Autodesk Inventor part; units mm, degrees
ref_plane "YZ Plane" through (0, 0, 0) normal (1, 0, 0) x (0, 1, 0)
ref_plane "XZ Plane" through (0, 0, 0) normal (0, 1, 0) x (-1, 0, 0)
ref_plane "XY Plane" through (0, 0, 0) normal (0, 0, 1) x (1, 0, 0)
sketch "Sketch1" plane through (0, 0, 0) normal (0, 0, 1) x (1, 0, 0)
  line L0 (-52.5, -20) -> (52.5, -20)
  line L1 (52.5, 20) -> (-52.5, 20)
  line L2 (-52.5, -20) -> (52.5, 20) construction
  line L3 (52.5, -20) -> (-52.5, 20) construction
  line L4 (-50, 17.5) -> (50, 17.5)
  line L5 (50, -17.5) -> (-50, -17.5)
  line L6 (-50, 17.5) -> (50, -17.5) construction
  line L7 (50, 17.5) -> (-50, -17.5) construction
  line L8 (60.5, 0) -> (60.5, 8)
  line L9 (60.5, 8) -> (52.5, 20)
  line L10 (60.5, 0) -> (60.5, -8)
  line L11 (60.5, -8) -> (52.5, -20)
  line L12 (50, -17.5) -> (56.5426, -7.6861)
  line L13 (56.5426, -7.6861) -> (56.5426, 7.6861)
  line L14 (56.5426, 7.6861) -> (50, 17.5)
  line L15 (0, 0) -> (0, 38.4543) construction
  line L16 (-60.5, 0) -> (-60.5, 8)
  line L17 (-60.5, 8) -> (-52.5, 20)
  line L18 (-60.5, 0) -> (-60.5, -8)
  line L19 (-60.5, -8) -> (-52.5, -20)
  line L20 (-50, -17.5) -> (-56.5426, -7.6861)
  line L21 (-56.5426, -7.6861) -> (-56.5426, 7.6861)
  line L22 (-56.5426, 7.6861) -> (-50, 17.5)
  dimension "d0" = 105
  dimension "d1" = 40
  dimension "d2" = 100
  dimension "d3" = 35
  dimension "d5" = 8
  dimension "d6" = 8
extrude "Extrusion1" add sketch "Sketch1" along normal blind 120
sketch "Sketch2" plane through (0, 0, 120) normal (0, 0, 1) x (1, 0, 0)
  line L0 (-56.5426, 7.6861) -> (-50, 17.5)
  line L1 (-50, 17.5) -> (50, 17.5)
  line L2 (50, 17.5) -> (56.5426, 7.6861)
  line L3 (56.5426, 7.6861) -> (56.5426, -7.6861)
  line L4 (56.5426, -7.6861) -> (50, -17.5)
  line L5 (50, -17.5) -> (-50, -17.5)
  line L6 (-50, -17.5) -> (-56.5426, -7.6861)
  line L7 (-56.5426, -7.6861) -> (-56.5426, 7.6861)
  point P0 (0, 0)
extrude "Extrusion2" add sketch "Sketch2" against normal blind 2.5
sketch "Sketch3" plane through (0, 0, 0) normal (0, 0, -1) x (-1, 0, 0)
  point P0 (0, 0)
fillet "Fillet1" radius 1 2 edges at (0, -17.5, 117.5) (0, 17.5, 117.5)
chamfer "Chamfer1" distance 5 angle 45 6 edges at (0, 20, 120) (-56.5, 14, 120) (-56.5, -14, 120) (0, -20, 120) (56.5, 14, 120) (56.5, -14, 120)
sketch "Sketch4" plane through (-52.5, -20, 0) normal (0, -1, 0) x (1, 0, 0)
  point P0 (52.5, 0)
sketch "Sketch5" plane through (0, 0, 0) normal (0, 0, -1) x (-1, 0, 0)
  line L0 (-50, 17.5) -> (50, 17.5)
  line L1 (-50, 17.5) -> (-50, 24.1033)
  line L2 (-50, 24.1033) -> (-71.4575, 13.1576)
  line L3 (-71.4575, 13.1576) -> (-66.6293, -23.8647)
  line L4 (-66.6293, -23.8647) -> (1.9313, -29.9815)
  line L5 (1.9313, -29.9815) -> (78.5389, -23.8647)
  line L6 (78.5389, -23.8647) -> (75.9786, 8.2013)
  line L7 (75.9786, 8.2013) -> (50, 28.9973)
  line L8 (50, 28.9973) -> (50, 17.5)
  point P0 (0, 0)
extrude "Extrusion3" cut sketch "Sketch5" against normal blind 120
sketch "Sketch6" plane through (50, 17.5, 0) normal (1, 0, 0) x (0, 0, -1)
  point P0 (0, -17.5)
sketch "Sketch7" plane through (0, 0, 0) normal (0, 0, -1) x (-1, 0, 0)
  line L0 (-50, 20) -> (50, 20) construction
  line L1 (0, 20) -> (48, 20) construction
  point P0 (0, 0)
  dimension "d17" = 48
sketch "Sketch8" plane through (0, 0, 0) normal (0, 0, -1) x (-1, 0, 0)
  line L0 (49, 24.3422) -> (51, 24.3422)
  line L1 (51, 24.3422) -> (51, 15.6578)
  line L2 (51, 15.6578) -> (49, 15.6578)
  line L3 (49, 15.6578) -> (49, 24.3422)
  line L4 (-50, 20) -> (50, 20)
  line L5 (49, 24.3422) -> (51, 15.6578) construction
  line L6 (51, 24.3422) -> (49, 15.6578) construction
  point P0 (0, 0)
  dimension "d18" = 2
extrude "Extrusion4" cut sketch "Sketch8" against normal blind 120
ref_plane "Work Plane1" through (0, 20, 0) normal (-1, 0, 0) x (0, -1, 0)
mirror "Mirror1" about plane through (0, 20, 0) normal (-1, 0, 0) of "Extrusion4"
sketch "Sketch9" plane through (49, 17.5, 0) normal (1, 0, 0) x (0, 0, -1)
  line L0 (-2.9947, 0) -> (-12.9947, 0)
  line L1 (-12.9947, 0) -> (-12.9947, -1.5)
  line L2 (-12.9947, -1.5) -> (-2.9947, -1.5)
  line L3 (-2.9947, -1.5) -> (-2.9947, 0)
  line L4 (-115, 2.5) -> (-100, 2.5)
  line L5 (-97.7055, -1.5) -> (-87.7055, -1.5)
  line L6 (-87.7055, -1.5) -> (-87.7055, 0)
  line L7 (-87.7055, 0) -> (-97.7055, 0)
  line L8 (-97.7055, 0) -> (-97.7055, -1.5)
  point P0 (0, -17.5)
  point P1 (0, 2.5)
  dimension "d21" = 10
  dimension "d22" = 1.5
  dimension "d23" = 15
  dimension "d24" = 10
extrude "Extrusion5" add sketch "Sketch9" along normal blind 2 and the other way blind 10
mirror "Mirror2" about plane through (0, 20, 0) normal (-1, 0, 0) of "Extrusion5"
properties part number "Frame2"
Verification items for the finished model (mm, model axes). Give positions to 0.01 mm unless a question says otherwise; leave off trailing zeros. Write each loop counter-clockwise with the first axis right and the second up, starting at its lowest first coordinate (ties: lowest second). Pieces come first, ordered by that corner, then holes. Notation, with made-up numbers: M -9.75,67 L 31.25,67 A18 cw 31.25,92 Z; hole C -9.5,-26 d11. An arc over 180 degrees is marked long. Put each result on its own line as item: value. Start each with the question number.
1. Section check A-A (x = 41.5). Record the cut outline in (y, z).
2. Section check B-B (y = 18.55). Record the cut outline in (x, z).
3. Draft check along X on faces 1 (the face through (49, 19, 58)), 2 (the face through (1, 17.5, 58)), 3 (the face through (-49, 19, 58)), 4 (the face through (-45, 16, 93)). Enter one of: +X half, -X half, draft (parallel to the pull), parting line (faces both ways), or undercut.
4. Scan lines: line 1 along X through (y, z) = (16.3, 11.5); line 2 along Y through (x, z) = (20, 5); line 3 along Z through (x, y) = (41, 16.4). Record each from-to range of solid material in increasing order. Write a range as [from, to].
5. Section check C-C (z = 41). Record the cut outline in (x, y), and give its area (3 significant figures).
6. Go/stop test with flat-tipped pins: pin 1 Ø1.6 at (x, y) = (47.5, 16.5) entering from -Z; pin 2 Ø1.6 at (x, y) = (-45.5, 17) entering from +Z; pin 3 Ø1.2 at (x, y) = (47.5, 16.5) entering from +Z. Record where each tip stops, or that it passes through.
Answer list:
1. outline: M 16,2.99 L 17.5,2.99 L 17.5,0 L 20,0 L 20,115 L 17.5,117.5 L 17.5,97.71 L 16,97.71 L 16,87.71 L 17.5,87.71 L 17.5,12.99 L 16,12.99 Z
2. outline: M -49,0 L 49,0 L 49,116.45 L -49,116.45 Z
3. face 1: +X half
3. face 2: undercut
3. face 3: -X half
3. face 4: draft
4. line 1: [-51, -39], [39, 51]
4. line 2: [17.5, 20]
4. line 3: [2.99, 12.99], [87.71, 97.71]
5. outline: M -49,17.5 L 49,17.5 L 49,20 L -49,20 Z
5. area: 245 mm2
6. pin 1: z = 2.99
6. pin 2: z = 117.5
6. pin 3: z = 97.71
